```python
from build123d import *

# Parameters (mm, degrees)
SKETCH5_R                  = 14
SKETCH5_R_2                = 12.5
RING_DEPTH                 = 1
TEETH_DEPTH                = 1
SCREW_BUMPS_DEPTH          = 1
SCREW_CLEARENCE_HOLE_REACH = 22.572
SKETCH8_R                  = 1.65
CIR_PAT_FOR_SCREWS_COUNT   = 4
CIR_PAT_TEETH_COUNT        = 5


with BuildPart() as part:
    # Sketch5 → ring (new body)
    with BuildSketch(Plane.XY):
        Circle(SKETCH5_R)
        Circle(SKETCH5_R_2, mode=Mode.SUBTRACT)
    extrude(amount=RING_DEPTH)

    # Sketch6 → teeth (add)
    with BuildSketch(Plane.XY):
        with BuildLine():
            Line((-3.75, 15.039531243), (-2.940974774, 14.45175732))
            ThreePointArc((-2.940974774, 14.45175732), (-2.093195964, 14.041639747), (-1.155683759, 13.952218284))
            ThreePointArc((-1.155683759, 13.952218284), (-2.148028374, 13.834231967), (-3.129428252, 13.645756806))
            Line((-3.129428252, 13.645756806), (-3.75, 15.039531243))
        make_face()
        with BuildLine():
            Line((3.75, 15.039531243), (3.129428252, 13.645756806))
            ThreePointArc((3.129428252, 13.645756806), (2.148028374, 13.834231967), (1.155683759, 13.952218284))
            ThreePointArc((1.155683759, 13.952218284), (2.093195964, 14.041639747), (2.940974774, 14.45175732))
            Line((2.940974774, 14.45175732), (3.75, 15.039531243))
        make_face()
    teeth = extrude(amount=TEETH_DEPTH)

    # Sketch7 → screw bumps (add)
    with BuildSketch(Plane.XY):
        with BuildLine():
            Line((4.928560895, 11.487353372), (4.928560895, 13.103789051))
            Line((4.928560895, 13.103789051), (-4.928560895, 13.103789051))
            Line((-4.928560895, 13.103789051), (-4.928560895, 11.487353372))
            ThreePointArc((-4.928560895, 11.487353372), (-3.62045714, 11.426586745), (-2.858565319, 10.361528592))
            ThreePointArc((-2.858565319, 10.361528592), (0, 7.95), (2.858565319, 10.361528592))
            ThreePointArc((2.858565319, 10.361528592), (3.62045714, 11.426586745), (4.928560895, 11.487353372))
        make_face()
    screw_bumps = extrude(amount=SCREW_BUMPS_DEPTH)

    # Sketch8 → screw clearence hole (cut, up to next)
    with BuildSketch(Plane.XY.offset(1), mode=Mode.PRIVATE) as screw_clearence_hole_sk1:
        with Locations((0, 10.85)):
            Circle(SKETCH8_R)
    screw_clearence_hole_tool1 = extrude(screw_clearence_hole_sk1.sketch, amount=-SCREW_CLEARENCE_HOLE_REACH, mode=Mode.PRIVATE) & part.part
    screw_clearence_hole = screw_clearence_hole_tool1.solids().sort_by_distance((0, 10.85, 1))[0]
    add(screw_clearence_hole, mode=Mode.SUBTRACT)

    # cir pat for screws: screw bumps, screw clearence hole ×4 about axis
    cir_pat_for_screws_axis = Axis((0, 0, 0), (0, 0, 1))
    add([screw_bumps.rotate(cir_pat_for_screws_axis, i * 360 / CIR_PAT_FOR_SCREWS_COUNT) for i in range(1, CIR_PAT_FOR_SCREWS_COUNT)])
    add([screw_clearence_hole.rotate(cir_pat_for_screws_axis, i * 360 / CIR_PAT_FOR_SCREWS_COUNT) for i in range(1, CIR_PAT_FOR_SCREWS_COUNT)], mode=Mode.SUBTRACT)

    # cir.pat. teeth: teeth ×5 about axis
    cir_pat_teeth_axis = Axis((0, 0, 0), (0, 0, 1))
    for i in range(1, CIR_PAT_TEETH_COUNT):
        add(teeth.rotate(cir_pat_teeth_axis, i * 360 / CIR_PAT_TEETH_COUNT))


solid = part.part
```
Geometry check sheet. Reference: the model listing, model coordinates, mm. A direction names the side the tool comes from. Coordinates: 2 decimals unless noted, no trailing zeros. Order: outer loops, then holes, each group sorted by start corner. A loop starts at its lowest first (then second) coordinate and runs counter-clockwise, first axis right, second up. Notation, with made-up numbers: (62, 1) - (94, 1) arc R27 cw to (94, 29) - close; hole circle Ø2 at (87.5, -3). An arc over 180 degrees is marked (long way). Answer as a JSON object with one key per item and string values. Group by question number.
Item 1: Tool access check on faces 4 (the face through (5.65, -13.64, 0.49)), 5 (the face through (-13.31, 4.34, 0.49)), 6 (the face through (13.994, 2.359, 0.493)), 7 (the face through (12.707, 6.343, 0.493)), 8 (the face through (-3.637, 11.436, 0.493)). Record the directions out of +Z, -Z, +X, -X, +Y, -Y that give a thin tool (end or side, any length) a straight path to the whole face; none if there is none.
Item 2: Sectioned sample at A-A, the plane y = 0. Record the cut outline in (x, z), and give its area (3 significant figures).
Item 3: Scan lines: probe 1 along X at (y, z) = (-1, 0.3); probe 2 along Y at (x, z) = (8.5, 0.8); probe 3 along X at (y, z) = (7.75, 0.45). Record each from-to range of solid material in increasing order.
Item 4: Sectioned sample at D-D, the plane z = 0.2. Give the number of separate pieces and of enclosed holes in the cut face, and give its area (3 significant figures).
Item 5: Draft check along Y on faces 1 (the face through (11.417, -3.604, 0.493)), 2 (the face through (-12.586, 7.711, 0.493)), 3 (the face through (9.959, -10.125, 0.493)). Enter one of: +Y half, -Y half, draft (parallel to the pull), parting line (faces both ways), or undercut.
Item 6: Sectioned sample at C-C, the plane y = -7. Record the cut outline in (x, z).
Resolved:
{
 "1": {"face 4": "+Z, -Z, -Y", "face 5": "+Z, -Z, -X", "face 6": "+Z, -Z, +X, +Y", "face 7": "+Z, -Z, +X", "face 8": "+Z, -Z"},
 "2": {"outline": "(-14, 0) - (-12.5, 0) - (-12.5, 1) - (-14, 1) - close; (-9.2, 0) - (-7.95, 0) - (-7.95, 1) - (-9.2, 1) - close; (7.95, 0) - (9.2, 0) - (9.2, 1) - (7.95, 1) - close; (12.5, 0) - (14, 0) - (14, 1) - (12.5, 1) - close", "area": "5.50 mm^2"},
 "3": {"probe 1": "-13.96 to -12.16, -9.54 to -8.13, 8.13 to 9.54, 12.16 to 13.96", "probe 2": "-11.12 to -9.17, -1.7 to 1.7, 9.17 to 11.12", "probe 3": "-12.99 to -12.63, -11.66 to -9.81, 9.81 to 11.66, 12.63 to 12.99"},
 "4": {"separate pieces": "1", "enclosed holes": "5", "area": "196 mm^2"},
 "5": {"face 1": "undercut", "face 2": "+Y half", "face 3": "-Y half"},
 "6": {"outline": "(-12.12, 0) - (-10.36, 0) - (-10.36, 1) - (-12.12, 1) - close; (10.36, 0) - (12.12, 0) - (12.12, 1) - (10.36, 1) - close"}
}
